Work out the finished part from the listing and answer in its coordinate system (mm). Face numbers are marked on the shaded views. A direction names the side the tool comes from. Coordinates: 2 decimals unless noted, no trailing zeros. Order: outer loops, then holes, each group sorted by start corner. A loop starts at its lowest first (then second) coordinate and runs counter-clockwise, first axis right, second up. Notation, with made-up numbers: (77, 62.5) -> (98, 62.5) arc R22 cw to (98, 82.5) -> close; hole circle Ø5 at (-21, 25). An arc over 180 degrees is marked (long way). Answer as CSV lines item,"result". Start each with the question number.
Item 1: Which of the six approach directions +Z, -Z, +X, -X, +Y, -Y give full straight-line access (tool end or side, diameter ignored) to the marked faces 4, 5 and 6?
Item 2: Section B-B (y = 3) is taken. Write down the section's boundary in (x, z), then the cut area to 3 significant figures.
Item 3: Section D-D (x = 0) is taken. Write down the section's boundary in (y, z), then the cut area to 4 significant figures.
Item 4: Section C-C (z = 0.75) is taken. Write down the section's boundary in (x, y).
Item 5: Each of these flat-tipped pins is pushed along its axis until it touches: pin 1 Ø4 at (x, y) = (-1, 8) entering from +Z; pin 2 Ø4 at (x, z) = (-2, 3.5) entering from -Y; pin 3 Ø2.5 at (x, z) = (-9, 0) entering from -Y; pin 4 Ø3 at (x, z) = (9, -1) entering from +Y. Where does it stop, or does it pass through?
Item 6: Straight lines are drawn through the part: L1, parallel to X at y = 9.3, z = 0; L2, parallel to Z at x = 9, y = 2.25; L3, parallel to X at y = 10, z = 2. For each, find the intervals that lie inside material, in ascending order.
Item 7: For a pull along X with two mould halves and no side action, classify the marked faces 1, 2 and 3 as pulls with the +X half, pulls with the -X half, needs draft (parallel to the pull), parting line crosses it, or undercut.
Item 8: Section A-A (x = 9) is taken. Write down the section's boundary in (y, z).
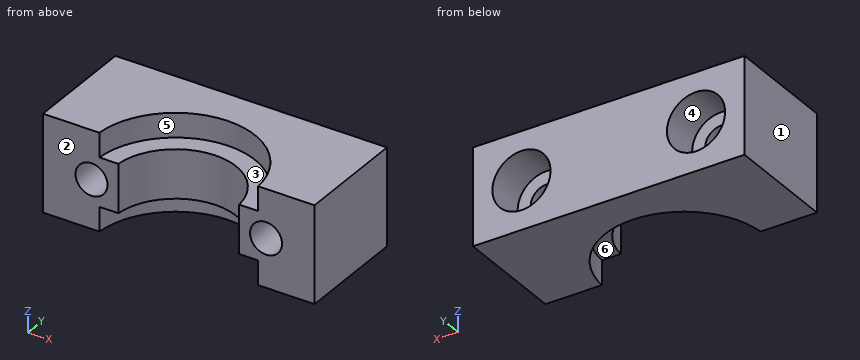
```python
from build123d import *

# Parameters (mm, degrees)
RESSALTO_EXTRUS_O1_DEPTH = 2.5
RESSALTO_EXTRUS_O2_DEPTH = 5
ESBO_O2_R                = 1.65
CORTE_EXTRUS_O1_DEPTH    = 15
ESBO_O4_R                = 3
CORTE_EXTRUS_O2_DEPTH    = 4


with BuildPart() as part:
    # Esboço1 → Ressalto-extrusão1 (new body, symmetric)
    with BuildSketch(Plane.XY):
        with BuildLine():
            Line((-6.229967897, 0.5), (-14, 0.5))
            Line((-14, 0.5), (-14, 12))
            Line((-14, 12), (14, 12))
            Line((14, 12), (14, 0.5))
            Line((14, 0.5), (6.229967897, 0.5))
            ThreePointArc((6.229967897, 0.5), (0, 6.25), (-6.229967897, 0.5))
        make_face()
    extrude(amount=RESSALTO_EXTRUS_O1_DEPTH, both=True)

    # Esboço3 → Ressalto-extrusão2 (add, symmetric)
    with BuildSketch(Plane.XY):
        with BuildLine():
            Line((-14, 12), (-14, 0.5))
            Line((-14, 0.5), (-8.184741902, 0.5))
            ThreePointArc((-8.184741902, 0.5), (0, 8.2), (8.184741902, 0.5))
            Line((8.184741902, 0.5), (14, 0.5))
            Line((14, 0.5), (14, 12))
            Line((14, 12), (-14, 12))
        make_face()
    extrude(amount=RESSALTO_EXTRUS_O2_DEPTH, both=True)

    # Esboço2 → Corte-extrusão1 (cut)
    with BuildSketch(Plane.XZ.offset(-0.5)):
        with Locations((-9, 0)):
            Circle(ESBO_O2_R)
        with Locations((9, 0)):
            Circle(ESBO_O2_R)
    extrude(amount=-CORTE_EXTRUS_O1_DEPTH, mode=Mode.SUBTRACT)

    # Esboço4 → Corte-extrusão2 (cut)
    with BuildSketch(Plane(origin=(0, 12, 0), x_dir=(1, 0, 0), z_dir=(0, 1, 0))):
        with Locations((-9, 0)):
            Circle(ESBO_O4_R)
        with Locations((9, 0)):
            Circle(ESBO_O4_R)
    extrude(amount=-CORTE_EXTRUS_O2_DEPTH, mode=Mode.SUBTRACT)


solid = part.part
```
Checked values:
1,face 4,"+Y"
1,face 5,"+Z, -Y"
1,face 6,"-Z, -Y"
2,outline,"(-14, -5) -> (-7.63, -5) -> (-7.63, -2.5) -> (-5.48, -2.5) -> (-5.48, 2.5) -> (-7.63, 2.5) -> (-7.63, 5) -> (-14, 5) -> close; (5.48, -2.5) -> (7.63, -2.5) -> (7.63, -5) -> (14, -5) -> (14, 5) -> (7.63, 5) -> (7.63, 2.5) -> (5.48, 2.5) -> close; hole circle Ø3.3 at (-9, 0); hole circle Ø3.3 at (9, 0)"
2,area,"132 mm^2"
3,outline,"(6.25, -2.5) -> (8.2, -2.5) -> (8.2, -5) -> (12, -5) -> (12, 5) -> (8.2, 5) -> (8.2, 2.5) -> (6.25, 2.5) -> close"
3,area,"47.75 mm^2"
4,outline,"(-14, 0.5) -> (-10.47, 0.5) -> (-10.47, 8) -> (-11.9, 8) -> (-11.9, 12) -> (-14, 12) -> close; (-7.53, 0.5) -> (-6.23, 0.5) arc R6.25 cw to (6.23, 0.5) -> (7.53, 0.5) -> (7.53, 8) -> (6.1, 8) -> (6.1, 12) -> (-6.1, 12) -> (-6.1, 8) -> (-7.53, 8) -> close; (10.47, 0.5) -> (14, 0.5) -> (14, 12) -> (11.9, 12) -> (11.9, 8) -> (10.47, 8) -> close"
5,pin 1,"stops at z = 5"
5,pin 2,"stops at y = 5.01"
5,pin 3,"passes through"
5,pin 4,"stops at y = 8"
6,L1,"x = -14 to -12, -6 to 6, 12 to 14"
6,L2,"z = -5 to -1.65, 1.65 to 5"
6,L3,"x = -14 to -11.24, -6.76 to 6.76, 11.24 to 14"
7,face 1,"pulls with the -X half"
7,face 2,"needs draft"
7,face 3,"undercut"
8,outline,"(0.5, -5) -> (12, -5) -> (12, -3) -> (8, -3) -> (8, -1.65) -> (0.5, -1.65) -> close; (0.5, 1.65) -> (8, 1.65) -> (8, 3) -> (12, 3) -> (12, 5) -> (0.5, 5) -> close"
